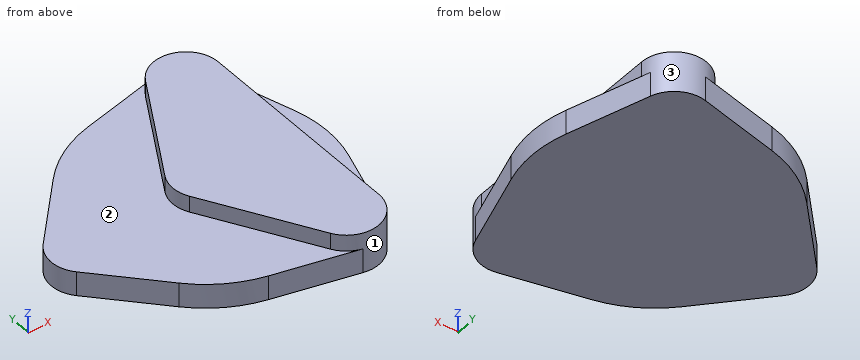
```python
from build123d import *

# Parameters (mm, degrees)
EXTRUDE_1_DEPTH = 6
EXTRUDE_2_DEPTH = 10


with BuildPart() as part:
    # 草圖1 → 填料-伸長1 (new body)
    with BuildSketch(Plane.XY):
        with BuildLine():
            Line((-22, 20.396078054), (-35.866666667, 5.438954148))
            ThreePointArc((-35.866666667, 5.438954148), (-38, 0), (-35.866666667, -5.438954148))
            Line((-35.866666667, -5.438954148), (-22, -20.396078054))
            ThreePointArc((-22, -20.396078054), (-15, -25.980762114), (-6.663521733, -29.25059791))
            Line((-6.663521733, -29.25059791), (13.223060871, -33.780921556))
            ThreePointArc((13.223060871, -33.780921556), (19, -32.908965344), (22.643605795, -28.341967408))
            Line((22.643605795, -28.341967408), (28.663521733, -8.854519856))
            ThreePointArc((28.663521733, -8.854519856), (30, 0), (28.663521733, 8.854519856))
            Line((28.663521733, 8.854519856), (22.643605795, 28.341967408))
            ThreePointArc((22.643605795, 28.341967408), (19, 32.908965344), (13.223060871, 33.780921556))
            Line((13.223060871, 33.780921556), (-6.663521733, 29.25059791))
            ThreePointArc((-6.663521733, 29.25059791), (-15, 25.980762114), (-22, 20.396078054))
        make_face()
    extrude(amount=EXTRUDE_1_DEPTH)

    # 草圖3 → 填料-伸長2 (add)
    with BuildSketch(Plane.XY):
        with BuildLine():
            Line((8.07179677, 29.980762114), (-6.92820323, 4))
            ThreePointArc((-6.92820323, 4), (-8, 0), (-6.92820323, -4))
            Line((-6.92820323, -4), (8.07179677, -29.980762114))
            ThreePointArc((8.07179677, -29.980762114), (17.070552361, -33.708168724), (23, -25.980762114))
            Line((23, -25.980762114), (23, 25.980762114))
            ThreePointArc((23, 25.980762114), (17.070552361, 33.708168724), (8.07179677, 29.980762114))
        make_face()
    extrude(amount=EXTRUDE_2_DEPTH)


solid = part.part
```
Geometry: final body of the model. Coordinates: model frame, mm. Face numbers are marked on the shaded views. A direction names the side the tool comes from. Coordinates: 2 decimals unless noted, no trailing zeros. Order: outer loops, then holes, each group sorted by start corner. A loop starts at its lowest first (then second) coordinate and runs counter-clockwise, first axis right, second up. Notation, with made-up numbers: (-29, -18.75) -> (15, -18.75) arc R23 cw to (15, 11.25) -> close; hole circle Ø8 at (24.5, 47). An arc over 180 degrees is marked (long way). Answer in a Markdown table with one row per item.
Item 1: Ray query, L1, parallel to Z at x = -28, y = 9; L2, parallel to X at y = 0, z = 6.75; L3, parallel to X at y = 8, z = 8.5. Return the intervals inside material, ascending.
Return value:
| item | result |
|---|---|
| L1 | z = 0 to 6 |
| L2 | x = -8 to 23 |
| L3 | x = -4.62 to 23 |
Item 2: Section C-C on x = 1. Output: boundary loops of the cut face in (y, z).
Return value:
| item | result |
|---|---|
| outline | (-31, 0) -> (31, 0) -> (31, 6) -> (17.73, 6) -> (17.73, 10) -> (-17.73, 10) -> (-17.73, 6) -> (-31, 6) -> close |
Item 3: Section A-A on z = 3.75. Output: boundary loops of the cut face in (x, y), plus the area to 3 significant figures.
Return value:
| item | result |
|---|---|
| outline | (-35.87, -5.44) -> (-22, -20.4) arc R30 ccw to (-6.66, -29.25) -> (13.22, -33.78) arc R8 ccw to (22.64, -28.34) -> (28.66, -8.85) arc R30 ccw to (28.66, 8.85) -> (22.64, 28.34) arc R8 ccw to (13.22, 33.78) -> (-6.66, 29.25) arc R30 ccw to (-22, 20.4) -> (-35.87, 5.44) arc R8 ccw to start |
| area | 3,280 mm² |
Item 4: Access query for the marked faces 1, 2 and 3. Directions: +Z, -Z, +X, -X, +Y, -Y. A direction counts if a zero-diameter tool reaches every point of the face in a straight line with its end or side. Return the directions, or none.
Return value:
| item | result |
|---|---|
| face 1 | +Z, -Y |
| face 2 | +Z, -X |
| face 3 | +Z, +Y |
Item 5: Section D-D on x = -12. Output: boundary loops of the cut face in (y, z).
Return value:
| item | result |
|---|---|
| outline | (-27.5, 0) -> (27.5, 0) -> (27.5, 6) -> (-27.5, 6) -> close |
Item 6: Section B-B on y = -19. Output: boundary loops of the cut face in (x, z).
Return value:
| item | result |
|---|---|
| outline | (-23.29, 0) -> (25.53, 0) -> (25.53, 6) -> (23, 6) -> (23, 10) -> (1.73, 10) -> (1.73, 6) -> (-23.29, 6) -> close |
Item 7: Contact query for flat-ended pins moving along their axis: P1, Ø3, axis at y = -9, z = 9, coming from the +X side; P2, Ø5, axis at x = -1.5, y = 8.5, coming from the -Z side; P3, Ø2, axis at x = -21.5, z = 8, coming from the +Y side; P4, Ø6, axis at y = -25.5, z = 1.5, coming from the -X side. Output: stop coordinate, or through.
Return value:
| item | result |
|---|---|
| P1 | stops at x = 23 |
| P2 | stops at z = 0 |
| P3 | passes through |
| P4 | stops at x = -19.84 |
